Geometry check sheet. Reference: the model listing, model coordinates, mm. Face numbers are marked on the shaded views. A direction names the side the tool comes from. Round coordinates to 2 decimals unless told otherwise and drop trailing zeros. Write each loop counter-clockwise with the first axis right and the second up, starting at its lowest first coordinate (ties: lowest second). Pieces come first, ordered by that corner, then holes. Notation, with made-up numbers: (48, 23.5) - (105, 23.5) arc R24 ccw to (105, 47.5) - close; hole circle Ø5 at (-8.75, 27.5). An arc over 180 degrees is marked (long way). One line per question, with ' | ' between items. Start each with the question number.
from build123d import *

# Parameters (mm, degrees)
BOX_W           = 17
BOX_H           = 38
BOX_DEPTH       = 20
SKETCH_R        = 7.66
SKETCH_W        = 8.5
SKETCH_H        = 8.5
POCKET_DEPTH    = 17.001
SKETCH005_R     = 1.52
POCKET001_DEPTH = 5
SKETCH006_R     = 1.68
POCKET002_DEPTH = 13
FILLET_R        = 7
CHAMFER_SIZE    = 2


with BuildPart() as part:
    # Box → Box (new body)
    with BuildSketch(Plane(origin=(0, 38, 0), x_dir=(1, 0, 0), z_dir=(0, 0, 1))):
        with Locations((8.5, 19)):
            Rectangle(BOX_W, BOX_H)
    extrude(amount=BOX_DEPTH)

    # Sketch → Pocket (cut, through all)
    with BuildSketch(Plane(origin=(17, 38, 0), x_dir=(0, 1, 0), z_dir=(1, 0, 0))):
        with Locations((19, 9.5)):
            Circle(SKETCH_R)
        with Locations((4.25, 15.75)):
            Rectangle(SKETCH_W, SKETCH_H)
        with Locations((33.75, 15.75)):
            Rectangle(SKETCH_W, SKETCH_H)
    extrude(amount=-POCKET_DEPTH, mode=Mode.SUBTRACT)

    # Sketch005 → Pocket001 (cut)
    with BuildSketch(Plane(origin=(0, 38, 20), x_dir=(1, 0, 0), z_dir=(0, 0, 1))):
        with Locations((8.5, 19)):
            Circle(SKETCH005_R)
    extrude(amount=-POCKET001_DEPTH, mode=Mode.SUBTRACT)

    # Sketch006 → Pocket002 (cut)
    with BuildSketch(Plane(origin=(0, 38, 0), x_dir=(1, 0, 0), z_dir=(0, 0, -1))):
        with Locations((8.5, -33)):
            Circle(SKETCH006_R)
        with Locations((8.5, -5)):
            Circle(SKETCH006_R)
    extrude(amount=-POCKET002_DEPTH, mode=Mode.SUBTRACT)

    # Fillet
    fillet_edges = [part.edges().sort_by_distance(p)[0] for p in [
        (8.5, 46.5, 20),
        (8.5, 67.5, 20),
    ]]
    fillet(fillet_edges, radius=FILLET_R)

    # Chamfer
    chamfer_edges = [part.edges().sort_by_distance(p)[0] for p in [
        (8.5, 38, 11.5),
        (8.5, 76, 11.5),
    ]]
    chamfer(chamfer_edges, length=CHAMFER_SIZE)


solid = part.part
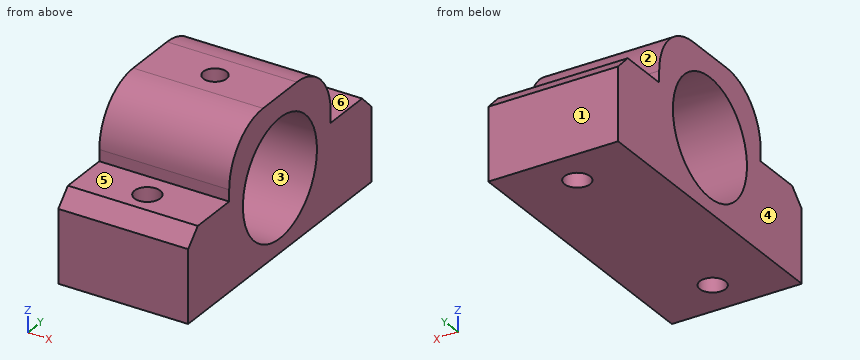
Q1. Draft check along Z on the marked faces 1, 2 and 3. Enter one of: pulls with the +Z half, pulls with the -Z half, needs draft (parallel to the pull), parting line crosses it, or undercut.
Q2. Set-up check for the marked faces 4, 5 and 6: record each of +Z, -Z, +X, -X, +Y, -Y from which the full face is reachable in a straight line by a thin tool's end or side.
Q3. Go/stop test with flat-tipped pins: P1, Ø1.2, axis at x = 5.5, z = 12, coming from the -Y side; P2, Ø7, axis at x = 5, y = 44.5, coming from the +Z side; P3, Ø1.5, axis at x = 8.5, z = 18, coming from the -Y side; P4, Ø2, axis at x = 8.5, y = 71, coming from the -Z side. Record where each tip stops, or that it passes through.
Q4. Section check A-A, the plane y = 57. Record the cut outline in (x, z).
Q5. Section check D-D, the plane y = 71. Record the cut outline in (x, z), then the cut area to 3 significant figures.
Q6. Section check B-B, the plane x = 3. Record the cut outline in (y, z), then the cut area to 3 significant figures.
Q7. Thickness scan on line 1 (X direction, y = 71, z = 4); line 2 (Y direction, x = 8.5, z = 7); line 3 (Y direction, x = 8.5, z = 8.5). Record the ranges inside material, lowest first.
Q8. Section check C-C, the plane z = 15. Record the cut outline in (x, y).
Result sheet:
1) face 1: needs draft | face 2: pulls with the +Z half | face 3: undercut
2) face 4: +Z, -Z, -X, +Y, -Y | face 5: +Z, +X, -X, -Y | face 6: +Z, +X, -X, +Y
3) P1: y = 39.9 | P2: z = 17.33 | P3: y = 47.94 | P4: through
4) outline: (0, 0) - (17, 0) - (17, 1.84) - (0, 1.84) - close; (0, 17.16) - (6.98, 17.16) - (6.98, 20) - (0, 20) - close; (10.02, 17.16) - (17, 17.16) - (17, 20) - (10.02, 20) - close
5) outline: (0, 0) - (6.82, 0) - (6.82, 11.5) - (0, 11.5) - close; (10.18, 0) - (17, 0) - (17, 11.5) - (10.18, 11.5) - close | area: 157 mm²
6) outline: (38, 0) - (76, 0) - (76, 9.5) - (74, 11.5) - (67.5, 11.5) - (67.5, 13) arc R7 ccw to (60.5, 20) - (53.5, 20) arc R7 ccw to (46.5, 13) - (46.5, 11.5) - (40, 11.5) - (38, 9.5) - close; hole circle Ø15.32 at (57, 9.5) | area: 406 mm²
7) line 1: 0 to 6.82, 10.18 to 17 | line 2: 38 to 41.32, 44.68 to 49.76, 64.24 to 69.32, 72.68 to 76 | line 3: 38 to 41.32, 44.68 to 49.41, 64.59 to 69.32, 72.68 to 76
8) outline: (0, 46.79) - (17, 46.79) - (17, 51.67) - (0, 51.67) - close; (0, 62.33) - (17, 62.33) - (17, 67.21) - (0, 67.21) - close
